```python
from build123d import *

# Parameters (mm, degrees)
F0_W     = 762
F0_H     = 609.6
F1_DEPTH = 19.05
F2_W     = 12.7
F2_H     = 12.7
F3_DEPTH = 762.001
F4_W     = 12.7
F4_H     = 12.7
F5_DEPTH = 609.601


with BuildPart() as f1:
    # F0 (on Front) → F1 (new body)
    with BuildSketch(Plane.XZ):
        with Locations((381, 304.8)):
            Rectangle(F0_W, F0_H)
    extrude(amount=F1_DEPTH)

    # F2 (on face) → F3 (cut, through all)
    with BuildSketch(Plane.YZ.offset(762)):
        with Locations((-6.35, 6.35)):
            Rectangle(F2_W, F2_H)
    extrude(amount=-F3_DEPTH, mode=Mode.SUBTRACT)

    # F4 (on face) → F5 (cut, through all)
    with BuildSketch(Plane.XY.offset(609.6)):
        with Locations((6.35, -6.35)):
            Rectangle(F4_W, F4_H)
    extrude(amount=-F5_DEPTH, mode=Mode.SUBTRACT)


solid = f1.part
```
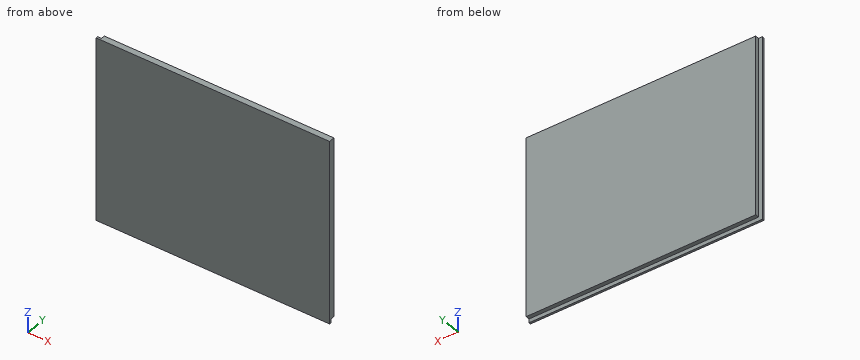
The listing builds one solid part. Answer for the finished solid, in the listing's coordinates (mm). Give positions to 0.01 mm unless a question says otherwise; leave off trailing zeros. Loops run counter-clockwise (first coordinate to the right, second up) from the corner with the lowest first, then second, coordinate; pieces in that order, holes last. Notation, with made-up numbers: M 64.5,88 L 83.5,88 A21 cw 83.5,126 Z; hole C 68.25,27 d9. An arc over 180 degrees is marked long. One line per item, written item: value.
1. Each of these flat-tipped pins is pushed along its axis until it touches: P1, Ø10, axis at x = 362, y = -7.5, coming from the -Z side; P2, Ø4, axis at y = -5, z = 254, coming from the -X side. Where does it stop, or does it pass through?
Found:
P1: z = 12.7
P2: x = 12.7
2. Find the intervals of material crossed by probe 1 along Z at (x, y) = (651, -9.75); probe 2 along X at (y, z) = (-9.5, 355.5), in increasing order.
Found:
probe 1: 12.7 to 609.6
probe 2: 12.7 to 762
3. Section A-A on y = -3.5 is taken. Determine the outline of the cut face in (x, z), plus the area to 3 significant figures.
Found:
outline: M 12.7,12.7 L 762,12.7 L 762,609.6 L 12.7,609.6 Z
area: 447,000 mm^2
